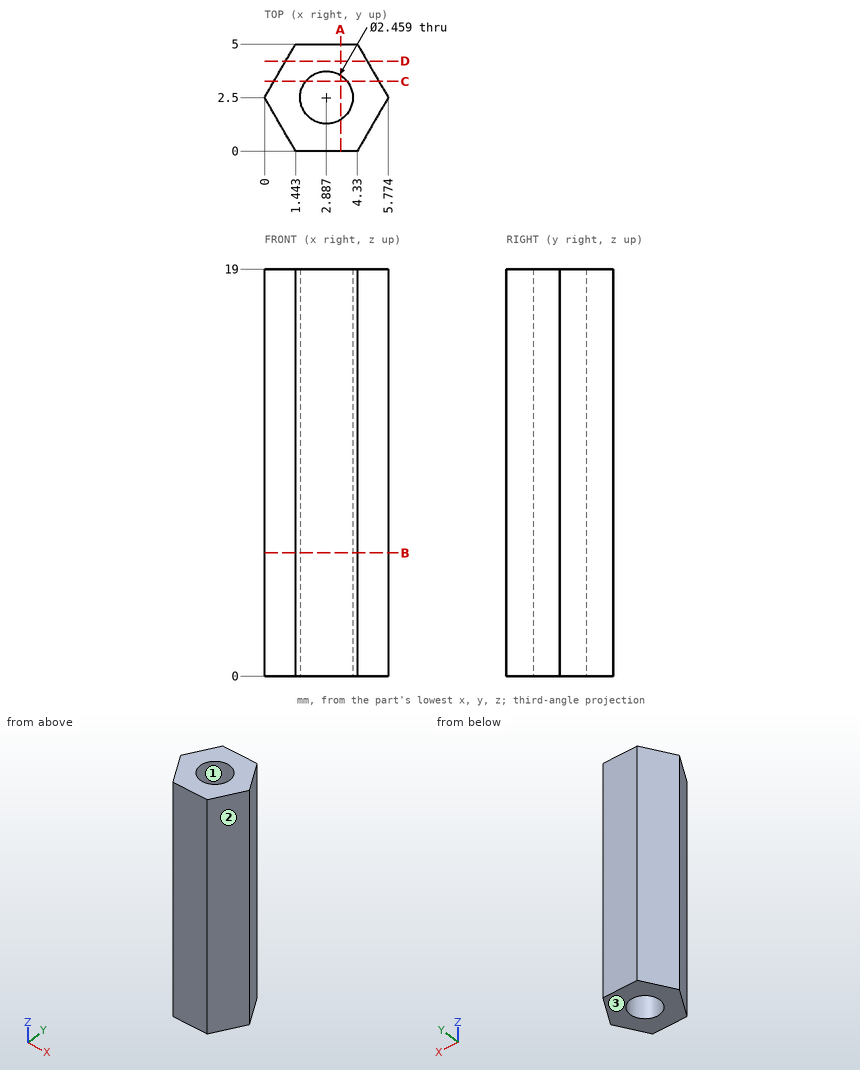
Check sheet for the drawn part. Datum: minimum x, y, z corner. Units: mm. Round coordinates to 2 decimals unless told otherwise and drop trailing zeros. Write each loop counter-clockwise with the first axis right and the second up, starting at its lowest first coordinate (ties: lowest second). Pieces come first, ordered by that corner, then holes. Notation, with made-up numbers: (33, -36.75) -> (90, -36.75) arc R23 cw to (90, 2.25) -> close; hole circle Ø9 at (-28, 4.5). An arc over 180 degrees is marked (long way). One line per item, written item: value. Start each with the question number.
(1) Cross-section at A-A, the plane x = 3.55. Record the cut outline in (y, z) (1 decimal).
(2) Cross-section at B-B, the plane z = 5.75. Record the cut outline in (x, y), and give its area (3 significant figures).
(3) Go/stop test with flat-tipped pins: pin 1 Ø1.5 at (y, z) = (3.5, 8) entering from -X (1 decimal); pin 2 Ø3 at (x, y) = (2.89, 2.5) entering from +Z. Record where each tip stops, or that it passes through.
(4) Draft check along X on the marked faces 1, 2 and 3. Enter one of: +X half, -X half, draft (parallel to the pull), parting line (faces both ways), or undercut.
(5) Cross-section at C-C, the plane y = 3.25. Record the cut outline in (x, z).
(6) Cross-section at D-D, the plane y = 4.2. Record the cut outline in (x, z), and give its area (3 significant figures).
(7) Scan lines: line 1 (X direction, y = 3.3, z = 4) (1 decimal); line 2 (X direction, y = 3.5, z = 6) (1 decimal); line 3 (Y direction, x = 1.85, z = 5.25). Record each from-to range of solid material in increasing order. Write a range as [from, to].
Answer:
1. outline: (0, 0) -> (1.5, 0) -> (1.5, 19) -> (0, 19) -> close; (3.5, 0) -> (5, 0) -> (5, 19) -> (3.5, 19) -> close
2. outline: (0, 2.5) -> (1.44, 0) -> (4.33, 0) -> (5.77, 2.5) -> (4.33, 5) -> (1.44, 5) -> close; hole circle Ø2.46 at (2.89, 2.5)
2. area: 16.9 mm²
3. pin 1: x = 0.1
3. pin 2: z = 19
4. face 1: undercut
4. face 2: +X half
4. face 3: draft
5. outline: (0.43, 0) -> (1.91, 0) -> (1.91, 19) -> (0.43, 19) -> close; (3.86, 0) -> (5.34, 0) -> (5.34, 19) -> (3.86, 19) -> close
6. outline: (0.98, 0) -> (4.79, 0) -> (4.79, 19) -> (0.98, 19) -> close
6. area: 72.4 mm²
7. line 1: [0.5, 2], [3.8, 5.3]
7. line 2: [0.6, 2.2], [3.6, 5.2]
7. line 3: [0, 1.84], [3.16, 5]
